```python
from build123d import *

# Parameters (mm, degrees)
CROQUIS1_W                         = 482.6
CROQUIS1_H                         = 62.738
BRIDA_BASE1_DEPTH                  = 1.524
BRIDA_DE_ARISTA1_STRIP_W           = 9.144
BRIDA_DE_ARISTA1_STRIP_H           = 1.524
BRIDA_DE_ARISTA1_STRIP_CUT_DEPTH   = 482.6
BRIDA_DE_ARISTA1_STRIP_2_W         = 9.144
BRIDA_DE_ARISTA1_STRIP_2_H         = 1.524
BRIDA_DE_ARISTA1_STRIP_CUT_2_DEPTH = 482.6
BRIDA_DE_ARISTA1_DEPTH             = 482.6
BRIDA_DE_ARISTA1_BEND_DEPTH        = 482.6
CROQUIS12_R                        = 3.9624
CORTAR_EXTRUIR1_DEPTH              = 58.166
CORTAR_EXTRUIR2_DEPTH              = 1.016
CORTAR_EXTRUIR2_DEPTH_BACK         = 3.048
CROQUIS13_W                        = 22.352
CROQUIS13_H                        = 16.002
CROQUIS14_W                        = 22.352
CROQUIS14_H                        = 16.002
CORTAR_EXTRUIR3_DEPTH              = 3.048
CROQUIS15_R                        = 3.937
CORTAR_EXTRUIR4_DEPTH              = 2.794


# Sheet-metal steps are written as plain solids
with BuildPart() as part:
    # Croquis1 → Brida base1 (new body)
    with BuildSketch(Plane.XY):
        Rectangle(CROQUIS1_W, CROQUIS1_H)
    extrude(amount=-BRIDA_BASE1_DEPTH)

    # Brida de arista1 strip (across the edge) → Brida de arista1 strip cut (cut)
    with BuildSketch(Plane(origin=(241.3, 31.369, 0), x_dir=(0, -1, 0), z_dir=(-1, 0, 0))):
        with Locations((-1.524, -0.762)):
            Rectangle(BRIDA_DE_ARISTA1_STRIP_W, BRIDA_DE_ARISTA1_STRIP_H)
    extrude(amount=BRIDA_DE_ARISTA1_STRIP_CUT_DEPTH, mode=Mode.SUBTRACT)

    # Brida de arista1 strip 2 (across the edge) → Brida de arista1 strip cut 2 (cut)
    with BuildSketch(Plane(origin=(-241.3, -31.369, 0), x_dir=(0, 1, 0), z_dir=(1, 0, 0))):
        with Locations((-1.524, -0.762)):
            Rectangle(BRIDA_DE_ARISTA1_STRIP_2_W, BRIDA_DE_ARISTA1_STRIP_2_H)
    extrude(amount=BRIDA_DE_ARISTA1_STRIP_CUT_2_DEPTH, mode=Mode.SUBTRACT)

    # Brida de arista1 section (across the edge) → Brida de arista1 (add)
    with BuildSketch(Plane(origin=(241.3, 31.369, 0), x_dir=(0, -1, 0), z_dir=(-1, 0, 0))):
        with BuildLine():
            Line((0, 1.524), (0, 14.478))
            Line((0, 14.478), (1.524, 14.478))
            Line((1.524, 14.478), (1.524, 1.524))
            ThreePointArc((1.524, 1.524), (1.970369265, 0.446369265), (3.048, 0))
            Line((3.048, 0), (3.048, -1.524))
            ThreePointArc((3.048, -1.524), (0.892738531, -0.631261469), (0, 1.524))
        make_face()
    extrude(amount=BRIDA_DE_ARISTA1_DEPTH)

    # Brida de arista1 section 2 (across the edge) → Brida de arista1 bend (add)
    with BuildSketch(Plane(origin=(-241.3, -31.369, 0), x_dir=(0, 1, 0), z_dir=(1, 0, 0))):
        with BuildLine():
            Line((0, 1.524), (0, 14.478))
            Line((0, 14.478), (1.524, 14.478))
            Line((1.524, 14.478), (1.524, 1.524))
            ThreePointArc((1.524, 1.524), (1.970369265, 0.446369265), (3.048, 0))
            Line((3.048, 0), (3.048, -1.524))
            ThreePointArc((3.048, -1.524), (0.892738531, -0.631261469), (0, 1.524))
        make_face()
    extrude(amount=BRIDA_DE_ARISTA1_BEND_DEPTH)

    # Croquis12 → Cortar-Extruir1 (cut)
    with BuildSketch(Plane.XY):
        with Locations((231.648, 16.383)):
            Circle(CROQUIS12_R)
        with Locations((231.648, 0.381)):
            Circle(CROQUIS12_R)
        with Locations((231.648, -15.367)):
            Circle(CROQUIS12_R)
        with Locations((-231.902, 16.383)):
            Circle(CROQUIS12_R)
        with Locations((-231.902, 0.381)):
            Circle(CROQUIS12_R)
        with Locations((-231.902, -15.367)):
            Circle(CROQUIS12_R)
    extrude(amount=-CORTAR_EXTRUIR1_DEPTH, mode=Mode.SUBTRACT)

    # Croquis13 → Cortar-Extruir2 (cut, two sides: drawn at the far end of the back side and taken through both)
    with BuildSketch(Plane(origin=(0, 31.369, 0), x_dir=(1, 0, 0), z_dir=(0, 1, 0)).offset(-CORTAR_EXTRUIR2_DEPTH_BACK)):
        with Locations((230.124, -6.477)):
            Rectangle(CROQUIS13_W, CROQUIS13_H)
        with Locations((-230.124, -6.477)):
            Rectangle(CROQUIS13_W, CROQUIS13_H)
    extrude(amount=CORTAR_EXTRUIR2_DEPTH + CORTAR_EXTRUIR2_DEPTH_BACK, mode=Mode.SUBTRACT)

    # Croquis14 → Cortar-Extruir3 (cut)
    with BuildSketch(Plane.XZ.offset(31.369)):
        with Locations((-230.124, 6.477)):
            Rectangle(CROQUIS14_W, CROQUIS14_H)
        with Locations((230.124, 6.477)):
            Rectangle(CROQUIS14_W, CROQUIS14_H)
    extrude(amount=-CORTAR_EXTRUIR3_DEPTH, mode=Mode.SUBTRACT)

    # Croquis15 → Cortar-Extruir4 (cut)
    with BuildSketch(Plane.XY):
        with Locations((-231.902, 30.6324)):
            Circle(CROQUIS15_R)
        with Locations((231.648, 30.6324)):
            Circle(CROQUIS15_R)
    extrude(amount=-CORTAR_EXTRUIR4_DEPTH, mode=Mode.SUBTRACT)


solid = part.part
```
For this review, take the finished solid that the model builds, in its own axes (mm). A direction names the side the tool comes from. Round coordinates to 2 decimals unless told otherwise and drop trailing zeros. Write each loop counter-clockwise with the first axis right and the second up, starting at its lowest first coordinate (ties: lowest second). Pieces come first, ordered by that corner, then holes. Notation, with made-up numbers: (41, -34.75) - (100, -34.75) arc R8 ccw to (100, -28.75) - close; hole circle Ø10 at (-26, 50). An arc over 180 degrees is marked (long way). Use CSV: the item, a comma, the result in double quotes.
1) The part is to be moulded in two halves that separate along X. For faces 1 (the flat face through (-3, -31.369, 8)), 2 (the cylindrical face through (-235.046, 13.972, -0.751)), say which applies: pulls with the +X half, pulls with the -X half, needs draft (parallel to the pull), parting line crosses it, or undercut.
Conclusion:
face 1,"needs draft"
face 2,"undercut"
2) For faces 3 (the flat face through (3, 29.845, 8)), 4 (the cylindrical face through (227.69, -15.19, -0.75)), list the 3-axis set-ups (+Z, -Z, +X, -X, +Y, -Y) from which the entire face can be reached by the end or side of a thin tool; tool diameter is ignored.
Conclusion:
face 3,"+Z, +X, -X"
face 4,"+Z, -Z"
3) Add section B-B on x = 35.5. Write out the cut boundary in (y, z) (3 decimals), and give its area (3 significant figures).
Conclusion:
outline,"(-31.369, 1.524) arc R3.048 ccw to (-28.321, -1.524) - (28.321, -1.524) arc R3.048 ccw to (31.369, 1.524) - (31.369, 14.478) - (29.845, 14.478) - (29.845, 1.524) arc R1.524 cw to (28.321, 0) - (-28.321, 0) arc R1.524 cw to (-29.845, 1.524) - (-29.845, 14.478) - (-31.369, 14.478) - close"
area,"137 mm^2"
4) Clearance check with flat-ended pins moving along their axes: pin 1 Ø1.5 at (y, z) = (30.5, 7) entering from -X; pin 2 Ø9 at (x, y) = (231.648, 16.383) entering from +Z; pin 3 Ø0.8 at (x, z) = (-225, -1) entering from +Y. State where each tip first meets the part, or that it passes through.
Conclusion:
pin 1,"stops at x = -218.95"
pin 2,"stops at z = 0"
pin 3,"stops at y = 28.32"
5) Add section A-A on z = 10.5. Write out the cut boundary in (x, y) (3 decimals).
Conclusion:
outline,"(-218.948, -31.369) - (218.948, -31.369) - (218.948, -29.845) - (-218.948, -29.845) - close; (-218.948, 29.845) - (218.948, 29.845) - (218.948, 31.369) - (-218.948, 31.369) - close"
6) Wall thickness on line 1 along Y through (x, z) = (182, 9.5) (3 decimals); line 2 along Z through (x, y) = (39, -15); line 3 along Z through (x, y) = (172.5, 29.5): over which ranges is each line inside the solid? List them lowest first. Write a range as from..to.
Conclusion:
line 1,"y = -31.369..-29.845, 29.845..31.369"
line 2,"z = -1.52..0"
line 3,"z = -1.29..0.56"
